from build123d import *

# Parameters (mm, degrees)
F3_D           = 10.71626
F3_DEPTH       = 38.1
F3_CSINK_D     = 15.875
F3_CSINK_ANGLE = 82
F3_TIP         = 3.2194893086
F5_D           = 10.71626
F5_DEPTH       = 191.008
F5_TIP         = 3.2194893086
F6_R           = 0.508


with BuildPart() as f1:
    # F0 (on Front) → F1 (revolve)
    with BuildSketch(Plane.XZ):
        Polygon((0, 28.2575), (0, 0), (228.6, 0), (228.6, 15.875), (88.646, 15.875), (35.56, 28.2575), align=None)
    revolve(axis=Axis((114.3, 0, 0), (1, 0, 0)))

    # F3
    with Locations(Plane.YZ.offset(228.6)):
        with Locations((0, 0)):
            CounterSinkHole(F3_D / 2, F3_CSINK_D / 2, depth=F3_DEPTH, counter_sink_angle=F3_CSINK_ANGLE)
            with Locations((0, 0, -(F3_DEPTH + F3_TIP / 2))):  # 118° drill point
                Cone(0, F3_D / 2, F3_TIP, mode=Mode.SUBTRACT)

    # F5
    with Locations(Plane(origin=(0, 0, 0), x_dir=(0, -1, 0), z_dir=(-1, 0, 0))):
        with Locations((0, 0)):
            Hole(F5_D / 2, depth=F5_DEPTH)
            with Locations((0, 0, -(F5_DEPTH + F5_TIP / 2))):  # 118° drill point
                Cone(0, F5_D / 2, F5_TIP, mode=Mode.SUBTRACT)

    # F6
    f6_edges = [f1.edges().sort_by_distance(p)[0] for p in [
        (0, 0, -28.2575),
        (35.56, 0, -28.2575),
        (88.646, 0, -15.875),
        (228.6, 0, -15.875),
    ]]
    fillet(f6_edges, radius=F6_R)


solid = f1.part
Part model, mm, in its own coordinate system. Give positions to 0.01 mm unless a question says otherwise; leave off trailing zeros. Write each loop counter-clockwise with the first axis right and the second up, starting at its lowest first coordinate (ties: lowest second). Pieces come first, ordered by that corner, then holes.
1) Pin check, flat tips, straight feed: pin 1 (17 mm diameter, centred on y = 0, z = 0, fed in from -X); pin 2 (1.5 mm diameter, centred on x = 37, y = -21, fed in from -Z); pin 3 (6.5 mm diameter, centred on y = 0, z = 0, fed in from +X); pin 4 (10 mm diameter, centred on x = 51, y = 0, fed in from +Z). Stop position of each tip, or through.
Resolved:
pin 1: stops at x = 0
pin 2: stops at z = -19.26
pin 3: passes through
pin 4: stops at z = 25.82
2) Cut at A-A on x = 169.5. Write the cut outline in (y, z) (3 decimals), then the cut area to 3 significant figures.
Resolved:
outline: circle Ø31.75 at (0, 0); hole circle Ø10.716 at (0, 0)
area: 702 mm2
3) Two-plate mould, pull along Z, no slides. Class faces 1 (the face through (225.78, 4.35, -3.34)), 2 (the face through (157.42, -4.77, 15.14)), 3 (the face through (228.6, 7, -7)): released by +Z, released by -Z, zero draft, split by the parting line, or undercut.
Resolved:
face 1: undercut
face 2: split by the parting line
face 3: zero draft
4) Probe L1, parallel to Z at x = 203, y = 0 (3 decimals); L2, parallel to Z at x = 68, y = 0. List the from-to ranges inside material, lowest first.
Resolved:
L1: z = -15.875 to -5.358, 5.358 to 15.875
L2: z = -20.69 to -5.36, 5.36 to 20.69
5) Cut at B-B on x = 21. Write the cut outline in (y, z) (1 decimal), then the cut area to 3 significant figures.
Resolved:
outline: circle Ø56.5 at (0, 0); hole circle Ø10.7 at (0, 0)
area: 2,420 mm2
